Design review of the part built by this model. Coordinates are the model's own, in mm. Coordinates: 2 decimals unless noted, no trailing zeros. Loops run counter-clockwise (first coordinate to the right, second up) from the corner with the lowest first, then second, coordinate; pieces in that order, holes last.
Q1. Wall thickness on probe 1 along Y at (x, z) = (-38, 0.7) (3 decimals); probe 2 along Y at (x, z) = (-20, 0.6) (3 decimals); probe 3 along X at (y, z) = (23, 0.4) (3 decimals): over which ranges is each line inside the solid? List them lowest first.
Q2. Add section A-A on z = 0.6. Give the boundary of the cut face in (x, y) (3 decimals), and give its area (3 significant figures).
Q3. Add section B-B on y = 14.5. Give the boundary of the cut face in (x, z) (3 decimals).
Q4. Add section C-C on x = -26. Give the boundary of the cut face in (y, z) (3 decimals).
```python
from build123d import *

# Parameters (mm, degrees)
SKETCH1_W           = 95.25
SKETCH1_H           = 107.95
SKETCH1_W_2         = 82.55
SKETCH1_H_2         = 95.25
BOSS_EXTRUDE1_DEPTH = 0.762


with BuildPart() as part:
    # Sketch1 → Boss-Extrude1 (new body)
    # profile 1 of 5: a face of its own
    with BuildSketch(Plane.XY):
        Rectangle(SKETCH1_W, SKETCH1_H)
        Rectangle(SKETCH1_W_2, SKETCH1_H_2, mode=Mode.SUBTRACT)
    # profile 2 of 5: a face of its own
    with BuildSketch(Plane.XY):
        Polygon((-2.801470588, 0), (-41.275, -47.625), (-41.275, 47.625), align=None)
    # profile 3 of 5: a face of its own
    with BuildSketch(Plane.XY):
        Polygon((0, 3.175), (-41.275, 47.625), (41.275, 47.625), align=None)
    # profile 4 of 5: a face of its own
    with BuildSketch(Plane.XY):
        Polygon((2.801470588, 0), (41.275, 47.625), (41.275, -47.625), align=None)
    # profile 5 of 5: a face of its own
    with BuildSketch(Plane.XY):
        Polygon((41.275, -47.625), (0, -3.175), (-41.275, -47.625), align=None)
    extrude(amount=BOSS_EXTRUDE1_DEPTH)


solid = part.part
```
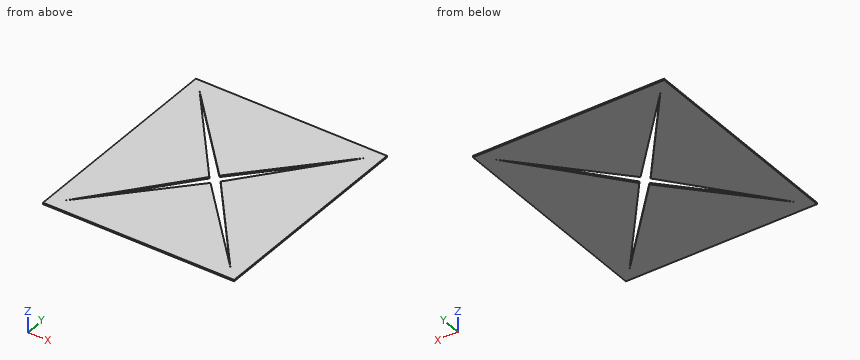
Entries:
1. probe 1: y = -53.975 to -44.098, -43.571 to 43.571, 44.098 to 53.975
1. probe 2: y = -53.975 to -24.713, -21.289 to 21.289, 24.713 to 53.975
1. probe 3: x = -47.625 to -21.382, -18.409 to 18.409, 21.382 to 47.625
2. outline: (-47.625, -53.975) - (47.625, -53.975) - (47.625, 53.975) - (-47.625, 53.975) - close; hole (-41.275, -47.625) - (0, -3.175) - (41.275, -47.625) - (2.801, 0) - (41.275, 47.625) - (0, 3.175) - (-41.275, 47.625) - (-2.801, 0) - close
2. area: 9,750 mm2
3. outline: (-47.625, 0) - (-14.515, 0) - (-14.515, 0.762) - (-47.625, 0.762) - close; (-10.516, 0) - (10.516, 0) - (10.516, 0.762) - (-10.516, 0.762) - close; (14.515, 0) - (47.625, 0) - (47.625, 0.762) - (14.515, 0.762) - close
4. outline: (-53.975, 0) - (-31.175, 0) - (-31.175, 0.762) - (-53.975, 0.762) - close; (-28.717, 0) - (28.717, 0) - (28.717, 0.762) - (-28.717, 0.762) - close; (31.175, 0) - (53.975, 0) - (53.975, 0.762) - (31.175, 0.762) - close
